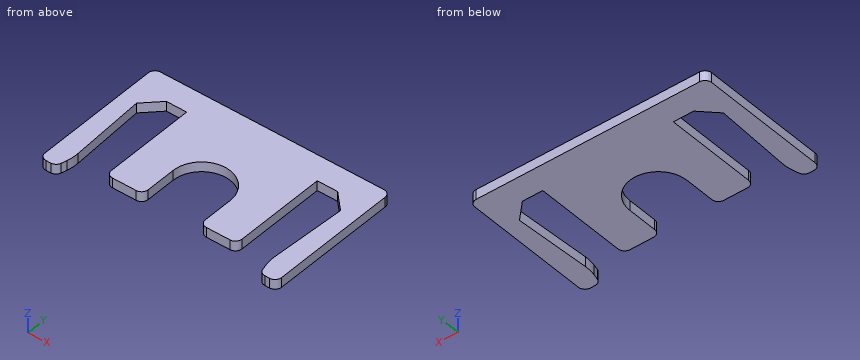
from build123d import *

# Parameters (mm, degrees)
BOSS_EXTRUDE1_DEPTH = 1.2
FILLET1_R           = 5
FILLET2_R           = 0.8


with BuildPart() as part:
    # Sketch1 → Boss-Extrude1 (new body)
    with BuildSketch(Plane.XY):
        with BuildLine():
            Line((-10.5, 0), (-12.5, -2))
            Line((-12.5, -2), (-12, -12))
            Line((-12, -12), (-12.5, -14))
            Line((-12.5, -14), (-14.5, -14))
            Line((-14.5, -14), (-14.5, 3))
            Line((-14.5, 3), (-12.5, 3))
            Line((-12.5, 3), (12.5, 3))
            Line((12.5, 3), (14.5, 3))
            Line((14.5, 3), (14.5, -14))
            Line((14.5, -14), (12.5, -14))
            Line((12.5, -14), (12, -12))
            Line((12, -12), (12.5, -2))
            Line((12.5, -2), (10.5, 0))
            Line((10.5, 0), (8, 0))
            Line((8, 0), (8, -12))
            Line((8, -12), (3.5, -12))
            Line((3.5, -12), (3.5, -7.5))
            ThreePointArc((3.5, -7.5), (0, -4), (-3.5, -7.5))
            Line((-3.5, -7.5), (-3.5, -12))
            Line((-3.5, -12), (-8, -12))
            Line((-8, -12), (-8, 0))
            Line((-8, 0), (-10.5, 0))
        make_face()
    extrude(amount=BOSS_EXTRUDE1_DEPTH)

    # Fillet1
    fillet1_edges = [part.edges().sort_by_distance(p)[0] for p in [
        (-12, -12, 0.6),
        (12, -12, 0.6),
    ]]
    fillet(fillet1_edges, radius=FILLET1_R)

    # Fillet2
    fillet2_edges = [part.edges().sort_by_distance(p)[0] for p in [
        (-12.5, -14, 0.6),
        (-14.5, -14, 0.6),
        (-14.5, 3, 0.6),
        (14.5, 3, 0.6),
        (14.5, -14, 0.6),
        (12.5, -14, 0.6),
        (8, -12, 0.6),
        (3.5, -12, 0.6),
        (-3.5, -12, 0.6),
        (-8, -12, 0.6),
    ]]
    fillet(fillet2_edges, radius=FILLET2_R)


solid = part.part
The listing builds one solid part. Answer for the finished solid, in the listing's coordinates (mm). Give positions to 0.01 mm unless a question says otherwise; leave off trailing zeros. Write each loop counter-clockwise with the first axis right and the second up, starting at its lowest first coordinate (ties: lowest second). Pieces come first, ordered by that corner, then holes. Notation, with made-up numbers: (19, -30.5) - (36, -30.5) arc R14 ccw to (36, -12.5) - close; hole circle Ø11 at (-28.75, -37.75). An arc over 180 degrees is marked (long way). One line per question, with ' | ' between items. Start each with the question number.
1. Section D-D, the plane x = 6.75 is taken. Determine the outline of the cut face in (y, z), then the cut area to 3 significant figures.
2. Section A-A, the plane y = -9 is taken. Determine the outline of the cut face in (x, z), then the cut area to 3 significant figures.
3. Straight lines are drawn through the part: line 1 (X direction, y = -8.5, z = 0.95) (3 decimals); line 2 (X direction, y = -0.5, z = 0.3); line 3 (X direction, y = -4.5, z = 0.5) (3 decimals). For each, find the intervals that lie inside material, in ascending order.
4. Section B-B, the plane y = -1.5 is taken. Determine the outline of the cut face in (x, z), then the cut area to 3 significant figures.
5. Given P1, Ø0.6, axis at x = -6.5, z = 0.5, coming from the -Y side, flat-ended and moving along its own axis, determine where the tip first touches the part or whether it passes through.
Result:
1) outline: (-12, 0) - (3, 0) - (3, 1.2) - (-12, 1.2) - close | area: 18.0 mm2
2) outline: (-14.5, 0) - (-12.15, 0) - (-12.15, 1.2) - (-14.5, 1.2) - close; (-8, 0) - (-3.5, 0) - (-3.5, 1.2) - (-8, 1.2) - close; (3.5, 0) - (8, 0) - (8, 1.2) - (3.5, 1.2) - close; (12.15, 0) - (14.5, 0) - (14.5, 1.2) - (12.15, 1.2) - close | area: 16.4 mm2
3) line 1: x = -14.5 to -12.175, -8 to -3.5, 3.5 to 8, 12.175 to 14.5 | line 2: x = -14.5 to -11, -8 to 8, 11 to 14.5 | line 3: x = -14.5 to -12.375, -8 to -1.803, 1.803 to 8, 12.375 to 14.5
4) outline: (-14.5, 0) - (-12, 0) - (-12, 1.2) - (-14.5, 1.2) - close; (-8, 0) - (8, 0) - (8, 1.2) - (-8, 1.2) - close; (12, 0) - (14.5, 0) - (14.5, 1.2) - (12, 1.2) - close | area: 25.2 mm2
5) P1: stops at y = -12
